Read the model definition and answer for the solid it produces. Units are mm, in the model's axes. A direction names the side the tool comes from. Give positions to 0.01 mm unless a question says otherwise; leave off trailing zeros. Write each loop counter-clockwise with the first axis right and the second up, starting at its lowest first coordinate (ties: lowest second). Pieces come first, ordered by that corner, then holes. Notation, with made-up numbers: (82, 50.25) -> (125, 50.25) arc R15 ccw to (125, 77.25) -> close; hole circle Ø3 at (-11, -29). An arc over 180 degrees is marked (long way). Write item = value, one per line.
from build123d import *

# Parameters (mm, degrees)
F4_D = 5


with BuildPart() as f1:
    # F0 (on Top) → F1 (revolve)
    with BuildSketch(Plane.XY):
        Polygon((0, 7.5), (0, 0), (30, 0), (30, 7), (25, 7), (25, 4.5), (20, 4.5), (20, 7.5), align=None)
    revolve(axis=Axis((15, 0, 0), (-1, 0, 0)))


with BuildPart() as f1_1:
    # F2: moved
    add(f1.part.moved(Location((0, 0, 7.5))))

    # F4 (through all)
    with Locations(Plane(origin=(0, 0, 0), x_dir=(1, 0, 0), z_dir=(0, 0, -1))):
        with Locations((7, 0)):
            Hole(F4_D / 2)


solid = f1_1.part
(1) The part is cut by section C-C on z = 1.25. Determine the outline of the cut face in (x, y), plus the area to 3 significant figures.
Checks:
outline = (0, -4.15) -> (20, -4.15) -> (20, 4.15) -> (0, 4.15) -> close; (25, -3.15) -> (30, -3.15) -> (30, 3.15) -> (25, 3.15) -> close; hole circle Ø5 at (7, 0)
area = 178 mm²
(2) The part is cut by section A-A on y = 0. Determine the outline of the cut face in (x, z), plus the area to 3 significant figures.
Checks:
outline = (0, 0) -> (4.5, 0) -> (4.5, 15) -> (0, 15) -> close; (9.5, 0) -> (20, 0) -> (20, 3) -> (25, 3) -> (25, 0.5) -> (30, 0.5) -> (30, 14.5) -> (25, 14.5) -> (25, 12) -> (20, 12) -> (20, 15) -> (9.5, 15) -> close
area = 340 mm²
(3) A tool of negligible diameter and unlimited length cuts with its end or side. For faces 1 (the flat face through (0, 0, 7)), 2 (the flat face through (20, 0.1, 12.4)), from which of +Z, -Z, +X, -X, +Y, -Y can it reach the whole face along a straight path? Write none if from no direction.
Checks:
face_1 = +Z, -Z, -X, +Y, -Y
face_2 = none
(4) The part is cut by section D-D on x = 7. Determine the outline of the cut face in (y, z).
Checks:
outline = (-2.5, 0.43) -> (-2.5, 14.57) arc R7.5 ccw to start; (2.5, 0.43) arc R7.5 ccw to (2.5, 14.57) -> close
(5) For a pull along X with two mould halves and no side action, classify faces 3 (the flat face through (25, 5, 7)), 4 (the flat face through (30, 0, 7)), 5 (the cylindrical face through (27.465, -1.517, 14.334)) as released by +X, released by -X, zero draft, split by the parting line, or undercut.
Checks:
face_3 = undercut
face_4 = released by +X
face_5 = zero draft
(6) Consider L1, parallel to X at y = 6.5, z = 5.5; L2, parallel to Z at x = 24, y = 0; L3, parallel to Y at x = 7, z = 9.5. Determine where each line is inside the solid, lowest interval first.
Checks:
L1 = 0 to 20, 25 to 30
L2 = 3 to 12
L3 = -7.23 to -2.5, 2.5 to 7.23
(7) The part is cut by section B-B on z = 7.5. Determine the outline of the cut face in (x, y).
Checks:
outline = (0, -7.5) -> (20, -7.5) -> (20, -4.5) -> (25, -4.5) -> (25, -7) -> (30, -7) -> (30, 7) -> (25, 7) -> (25, 4.5) -> (20, 4.5) -> (20, 7.5) -> (0, 7.5) -> close; hole circle Ø5 at (7, 0)
(8) Given P1, Ø4, axis at x = 7, y = 0, coming from the -Z side; P2, Ø4, axis at x = 4.5, z = 1.5, coming from the -Y side; P3, Ø1.5, axis at x = 11.5, y = 3.5, coming from the -Z side; P4, Ø4, axis at x = 8.5, y = -3.5, coming from the +Z side, each flat-ended and moving along its own axis, determine where each tip first touches the part or whether it passes through.
Checks:
P1 = through
P2 = -6.34
P3 = 0.52
P4 = 14.84
